```python
from build123d import *

# Parameters (mm, degrees)
BOSS_EXTRUDE1_DEPTH = 5
BOSS_EXTRUDE2_DEPTH = 2
SKETCH10_W          = 10
SKETCH10_H          = 5
BOSS_EXTRUDE7_DEPTH = 30
SKETCH11_R          = 3
BOSS_EXTRUDE8_DEPTH = 50


with BuildPart() as part:
    # Sketch1 → Boss-Extrude1 (new body)
    with BuildSketch(Plane(origin=(0, 0, 0), x_dir=(1, 0, 0), z_dir=(0, 1, 0))):
        Polygon((-15, 15), (-25, 15), (-25, -15), (25, -15), (25, 15), (15, 15), (13.266499161, 7), (-13.266499161, 7), align=None)
    extrude(amount=BOSS_EXTRUDE1_DEPTH)

    # Sketch4 → Boss-Extrude2 (add)
    with BuildSketch(Plane.XZ):
        with BuildLine():
            Line((13.266499161, 7), (-13.266499161, 7))
            ThreePointArc((-13.266499161, 7), (-15, 0), (-13.266499161, -7))
            Line((-13.266499161, -7), (13.266499161, -7))
            ThreePointArc((13.266499161, -7), (14.560176637, -3.605725487), (15, 0))
            ThreePointArc((15, 0), (14.560176637, 3.605725487), (13.266499161, 7))
        make_face()
    extrude(amount=BOSS_EXTRUDE2_DEPTH)

    # Sketch10 → Boss-Extrude7 (add)
    with BuildSketch(Plane.XY.offset(15)):
        with Locations((-20, 7.5)):
            Rectangle(SKETCH10_W, SKETCH10_H)
        Polygon((-15, 5), (-10, 10), (-15, 10), align=None)
        Polygon((15, 5), (10, 10), (15, 10), align=None)
        with Locations((20, 7.5)):
            Rectangle(SKETCH10_W, SKETCH10_H)
    extrude(amount=-BOSS_EXTRUDE7_DEPTH)

    # Sketch11 → Boss-Extrude8 (add)
    with BuildSketch(Plane(origin=(25, 0, 0), x_dir=(0, 0, -1), z_dir=(1, 0, 0))):
        with BuildLine():
            Line((-7, -7), (-7, -2))
            Line((-7, -2), (7, -2))
            Line((7, -2), (7, -7))
            ThreePointArc((7, -7), (0, -14), (-7, -7))
        make_face()
        with Locations((0, -7)):
            Circle(SKETCH11_R, mode=Mode.SUBTRACT)
    extrude(amount=-BOSS_EXTRUDE8_DEPTH)


solid = part.part
```
Work out the finished part from the listing and answer in its coordinate system (mm). A direction names the side the tool comes from. Coordinates: 2 decimals unless noted, no trailing zeros. Order: outer loops, then holes, each group sorted by start corner. A loop starts at its lowest first (then second) coordinate and runs counter-clockwise, first axis right, second up. Notation, with made-up numbers: (42.5, 1) - (70.5, 1) arc R12 ccw to (70.5, 15) - close; hole circle Ø1 at (10, 4). An arc over 180 degrees is marked (long way). Answer as a JSON object with one key per item and string values.
1. Each of these flat-tipped pins is pushed along its axis until it touches: P1, Ø9, axis at x = -2.5, z = 1, coming from the +Y side; P2, Ø1, axis at x = -14.5, z = -10.5, coming from the -Y side; P3, Ø1, axis at x = 19, y = -6.5, coming from the +Z side. Where does it stop, or does it pass through?
Output values:
{"P1": "stops at y = 5", "P2": "stops at y = 0", "P3": "stops at z = 7"}
2. Find section C-C on z = 8. Determine the outline of the cut face in (x, y), plus the area to 3 significant figures.
Output values:
{"outline": "(-25, 0) - (25, 0) - (25, 10) - (10, 10) - (15, 5) - (-15, 5) - (-10, 10) - (-25, 10) - close", "area": "375 mm²"}
3. A tool of negligible diameter and unlimited length cuts with its end or side. For faces 4 (the face through (-15, -1, 0)), 5 (the face through (13, 7, 0)), 6 (the face through (0, -2, -7)), 7 (the face through (25, 5, 0)), from which of +Z, -Z, +X, -X, +Y, -Y can it reach the whole face along a straight path? Write none if from no direction.
Output values:
{"face 4": "-X", "face 5": "+Z, -Z", "face 6": "-Z, -Y", "face 7": "+Z, -Z, +X, +Y, -Y"}
4. Find section D-D on z = -1.5. Determine the outline of the cut face in (x, y), plus the area to 3 significant figures.
Output values:
{"outline": "(-25, -13.84) - (25, -13.84) - (25, -9.6) - (-25, -9.6) - close; (-25, -4.4) - (25, -4.4) - (25, -2) - (14.92, -2) - (14.92, 0) - (25, 0) - (25, 10) - (10, 10) - (15, 5) - (-15, 5) - (-10, 10) - (-25, 10) - (-25, 0) - (-14.92, 0) - (-14.92, -2) - (-25, -2) - close", "area": "767 mm²"}
5. Consider line 1 (Y direction, x = 19, z = 0.75); line 2 (Y direction, x = 3, z = 0); line 3 (Z direction, x = -4, y = 4). Determine where each line is inside the solid, lowest interval first.
Output values:
{"line 1": "y = -13.96 to -9.9, -4.1 to -2, 0 to 10", "line 2": "y = -14 to -10, -4 to 5", "line 3": "z = -7 to 15"}
6. Find section A-A on x = 12. Determine the outline of the cut face in (y, z), plus the area to 3 significant figures.
Output values:
{"outline": "(-7, -7) - (5, -7) - (5, 15) - (0, 15) - (0, 7) - (-7, 7) arc R7 ccw to start; (8, -15) - (10, -15) - (10, 15) - (8, 15) - close; hole circle Ø6 at (-7, 0)", "area": "317 mm²"}
7. Find section B-B on y = 5.75. Determine the outline of the cut face in (x, z), plus the area to 3 significant figures.
Output values:
{"outline": "(-25, -15) - (-14.25, -15) - (-14.25, 15) - (-25, 15) - close; (14.25, -15) - (25, -15) - (25, 15) - (14.25, 15) - close", "area": "645 mm²"}
8. The mould has two halves that part along X. Classify faces 1 (the face through (0, 5, 3)), 2 (the face through (0, -4, 7)), 3 (the face through (25, -8, 3)): +X half, -X half, draft (parallel to the pull), parting line (faces both ways), or undercut.
Output values:
{"face 1": "undercut", "face 2": "draft", "face 3": "+X half"}
